Here's how the part is built. I have some questions about the finished solid (model axes, mm). Face numbers are marked on the shaded views. Coordinates: 2 decimals unless noted, no trailing zeros. Order: outer loops, then holes, each group sorted by start corner. A loop starts at its lowest first (then second) coordinate and runs counter-clockwise, first axis right, second up. Notation, with made-up numbers: (-14, 49.25) - (-6, 49.25) arc R26 cw to (-6, 85.25) - close; hole circle Ø9 at (14.25, 31.5). An arc over 180 degrees is marked (long way). Answer in a Markdown table with one row per item. Add a question column.
Item 1: I want a section at B-B (y = 0). Please give me the cut outline in (x, z).
Item 2: Thinking about a two-plate mould opening in Y: for the marked faces 1, 2 and 3, which applies, +Y half, -Y half, draft (parallel to the pull), parting line (faces both ways), or undercut?
Item 3: I want a section at A-A (x = 0). Please give me the cut outline in (y, z), plus the area to 3 significant figures.
Item 4: I want a section at C-C (x = -31.5). Please give me the cut outline in (y, z).
Item 5: Will these pins go through, and if not, where does the flat tip stop? pin 1 Ø2 at (x, z) = (16.5, -6.5) entering from +Y; pin 2 Ø2.5 at (x, y) = (-38.97, 22.5) entering from +Z; pin 3 Ø3.5 at (x, y) = (0, -45) entering from -Z; pin 4 Ø6 at (x, z) = (-11, -20.5) entering from +Y.
Item 6: If I drill on line 1 along Y through (x, z) = (0, -23.8); line 2 along Y through (x, z) = (0, -12.5); line 3 along Z through (x, y) = (28, 32), over which ranges is the centre line in solid material (lowest first)? Write a range as from..to.
Item 7: I want a section at D-D (z = -20.75). Please give me the cut outline in (x, y).
```python
from build123d import *

# Parameters (mm, degrees)
ESQUISSE1_R        = 40.4
ESQUISSE1_R_2      = 40
BOSS_EXTRU_1_DEPTH = 25
BOSS_EXTRU_2_START = -2
ESQUISSE2_R        = 50
ESQUISSE2_R_2      = 1.6
ESQUISSE2_R_3      = 40
BOSS_EXTRU_2_DEPTH = 2


with BuildPart() as part:
    # Esquisse1 → Boss.-Extru.1 (new body)
    with BuildSketch(Plane.XY):
        Circle(ESQUISSE1_R)
        Circle(ESQUISSE1_R_2, mode=Mode.SUBTRACT)
    extrude(amount=-BOSS_EXTRU_1_DEPTH)

    # Esquisse2 → Boss.-Extru.2 (add)
    with BuildSketch(Plane(origin=(0, 0, -25), x_dir=(-1, 0, 0), z_dir=(0, 0, -1)).offset(BOSS_EXTRU_2_START)):
        Circle(ESQUISSE2_R)
        with Locations((-38.97114317, 22.5)):
            Circle(ESQUISSE2_R_2, mode=Mode.SUBTRACT)
        with Locations((38.97114317, 22.5)):
            Circle(ESQUISSE2_R_2, mode=Mode.SUBTRACT)
        with Locations((0, -45)):
            Circle(ESQUISSE2_R_2, mode=Mode.SUBTRACT)
        with Locations(Location((0, 0, 0), (0, 0, 180))):
            Circle(ESQUISSE2_R_3, mode=Mode.SUBTRACT)
    extrude(amount=BOSS_EXTRU_2_DEPTH)


solid = part.part
```
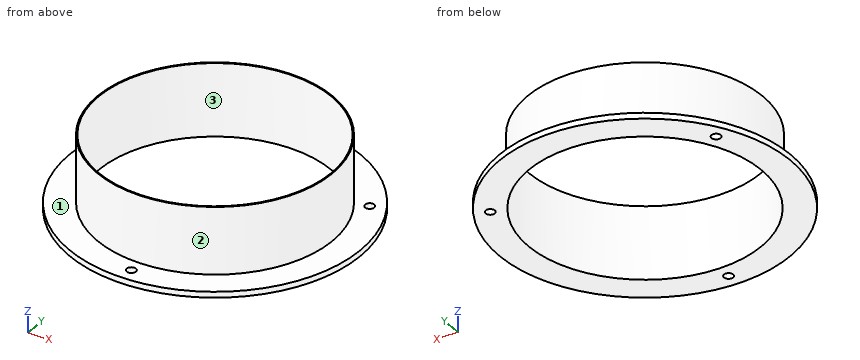
Values follow:
| question | item | result |
|---|---|---|
| 1 | outline | (-50, -25) - (-40, -25) - (-40, 0) - (-40.4, 0) - (-40.4, -23) - (-50, -23) - close; (40, -25) - (50, -25) - (50, -23) - (40.4, -23) - (40.4, 0) - (40, 0) - close |
| 2 | face 1 | draft |
| 2 | face 2 | parting line |
| 2 | face 3 | undercut |
| 3 | outline | (-50, -25) - (-46.6, -25) - (-46.6, -23) - (-50, -23) - close; (-43.4, -25) - (-40, -25) - (-40, 0) - (-40.4, 0) - (-40.4, -23) - (-43.4, -23) - close; (40, -25) - (50, -25) - (50, -23) - (40.4, -23) - (40.4, 0) - (40, 0) - close |
| 3 | area | 52.0 mm^2 |
| 4 | outline | (-38.83, -25) - (-24.65, -25) - (-24.65, 0) - (-25.3, 0) - (-25.3, -23) - (-38.83, -23) - close; (24.65, -25) - (38.83, -25) - (38.83, -23) - (25.3, -23) - (25.3, 0) - (24.65, 0) - close |
| 5 | pin 1 | stops at y = 37.31 |
| 5 | pin 2 | passes through |
| 5 | pin 3 | stops at z = -25 |
| 5 | pin 4 | stops at y = 49.12 |
| 6 | line 1 | y = -50..-46.6, -43.4..-40, 40..50 |
| 6 | line 2 | y = -40.4..-40, 40..40.4 |
| 6 | line 3 | z = -25..-23 |
| 7 | outline | circle Ø80.8 at (0, 0); hole circle Ø80 at (0, 0) |
